Part print with two shaded views. Sizes in mm from the minimum x, y, z corner. Give positions to 0.01 mm unless a question says otherwise; leave off trailing zeros. Write each loop counter-clockwise with the first axis right and the second up, starting at its lowest first coordinate (ties: lowest second). Pieces come first, ordered by that corner, then holes. Notation, with made-up numbers: (81.5, 14) -> (105.5, 14) arc R15 ccw to (105.5, 22) -> close; hole circle Ø7 at (-29.75, 87). An arc over 180 degrees is marked (long way). Answer in a Markdown table with one row per item. Add a question column.
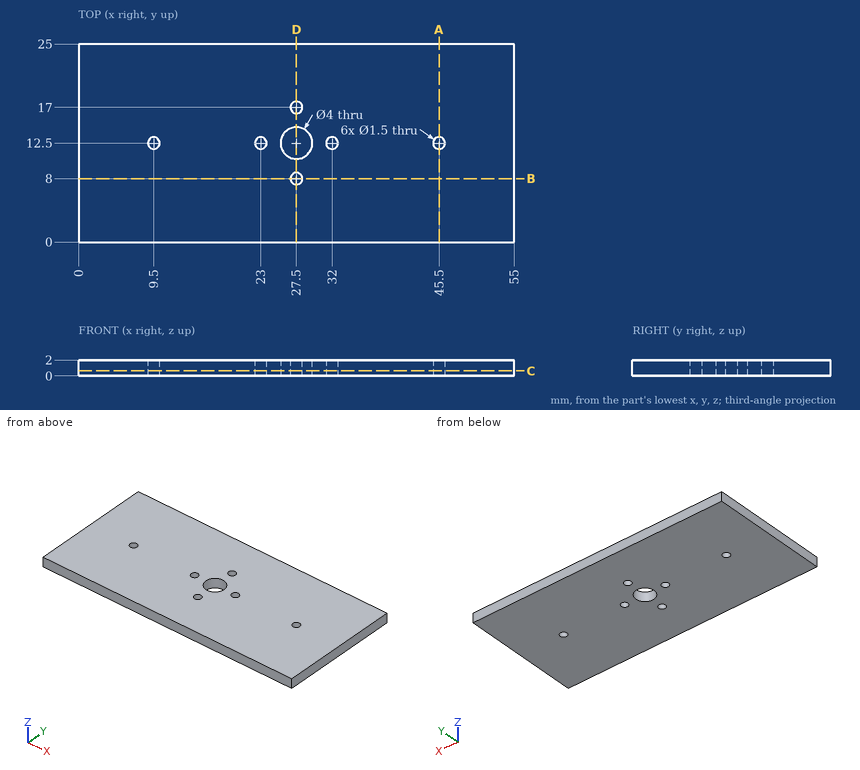
Item 1: Slice it at D-D, the plane x = 27.5. List the corners of the cut face in (y, z), then the cut area to 3 significant figures.
Item 2: Probe L1, parallel to Y at x = 27.5, z = 0.4; L2, parallel to Y at x = 45.5, z = 1.1; L3, parallel to Y at x = 46, z = 0.5. List the from-to ranges inside material, lowest first. Write a range as from..to.
Item 3: Slice it at C-C, the plane z = 0.65. List the corners of the cut face in (x, y).
Item 4: Slice it at A-A, the plane x = 45.5. List the corners of the cut face in (y, z), then the cut area to 3 significant figures.
Item 5: Slice it at B-B, the plane y = 8. List the corners of the cut face in (x, z), then the cut area to 3 significant figures.
Answer key:
| question | item | result |
|---|---|---|
| 1 | outline | (0, 0) -> (7.25, 0) -> (7.25, 2) -> (0, 2) -> close; (8.75, 0) -> (10.5, 0) -> (10.5, 2) -> (8.75, 2) -> close; (14.5, 0) -> (16.25, 0) -> (16.25, 2) -> (14.5, 2) -> close; (17.75, 0) -> (25, 0) -> (25, 2) -> (17.75, 2) -> close |
| 1 | area | 36.0 mm² |
| 2 | L1 | y = 0..7.25, 8.75..10.5, 14.5..16.25, 17.75..25 |
| 2 | L2 | y = 0..11.75, 13.25..25 |
| 2 | L3 | y = 0..11.94, 13.06..25 |
| 3 | outline | (0, 0) -> (55, 0) -> (55, 25) -> (0, 25) -> close; hole circle Ø1.5 at (9.5, 12.5); hole circle Ø1.5 at (23, 12.5); hole circle Ø4 at (27.5, 12.5); hole circle Ø1.5 at (27.5, 8); hole circle Ø1.5 at (27.5, 17); hole circle Ø1.5 at (32, 12.5); hole circle Ø1.5 at (45.5, 12.5) |
| 4 | outline | (0, 0) -> (11.75, 0) -> (11.75, 2) -> (0, 2) -> close; (13.25, 0) -> (25, 0) -> (25, 2) -> (13.25, 2) -> close |
| 4 | area | 47.0 mm² |
| 5 | outline | (0, 0) -> (26.75, 0) -> (26.75, 2) -> (0, 2) -> close; (28.25, 0) -> (55, 0) -> (55, 2) -> (28.25, 2) -> close |
| 5 | area | 107 mm² |
